```python
from build123d import *

# Parameters (mm, degrees)
EXTRUDE_THIN1_DEPTH = 635
FILLET1_R           = 1.27


with BuildPart() as part:
    # Sketch1 → Extrude-Thin1 (new body)
    with BuildSketch(Plane.XY):
        with BuildLine():
            Line((0, 0), (-15.875, 0))
            Line((-15.875, 0), (-15.875, 3.175))
            Line((-15.875, 3.175), (-19.05, 3.175))
            ThreePointArc((-19.05, 3.175), (-20.540376263, 7.805172974), (-24.451827217, 10.69658692))
            ThreePointArc((-24.451827217, 10.69658692), (-28.805679852, 14.276302994), (-29.685414913, 19.84375))
            Line((-29.685414913, 19.84375), (-32.860414913, 19.84375))
            Line((-32.860414913, 19.84375), (-32.860414913, 24.60625))
            Line((-32.860414913, 24.60625), (-36.494039614, 24.60625))
            ThreePointArc((-36.494039614, 24.60625), (-43.039469794, 22.912442068), (-47.941664913, 18.25625))
            Line((-47.941664913, 18.25625), (-56.672914913, 18.25625))
            Line((-56.672914913, 18.25625), (-56.672914913, 44.351036989))
            ThreePointArc((-56.672914913, 44.351036989), (-59.143520033, 43.316980719), (-60.876574207, 41.275))
            ThreePointArc((-60.876574207, 41.275), (-64.274926573, 48.035607826), (-63.5, 55.5625))
            Line((-63.5, 55.5625), (-34.925, 55.5625))
            Line((-34.925, 55.5625), (-34.925, 54.2925))
            Line((-34.925, 54.2925), (-62.614600616, 54.2925))
            ThreePointArc((-62.614600616, 54.2925), (-63.088488589, 48.638883567), (-60.958941974, 43.380273504))
            ThreePointArc((-60.958941974, 43.380273504), (-58.440775835, 45.159436942), (-55.402914913, 45.686679074))
            Line((-55.402914913, 45.686679074), (-55.402914913, 19.52625))
            Line((-55.402914913, 19.52625), (-48.62569758, 19.52625))
            ThreePointArc((-48.62569758, 19.52625), (-43.340564736, 24.19276788), (-36.494039614, 25.87625))
            Line((-36.494039614, 25.87625), (-31.590414913, 25.87625))
            Line((-31.590414913, 25.87625), (-31.590414913, 21.11375))
            Line((-31.590414913, 21.11375), (-27.922084416, 21.11375))
            ThreePointArc((-27.922084416, 21.11375), (-28.061990954, 15.63278224), (-24.046119572, 11.900040827))
            ThreePointArc((-24.046119572, 11.900040827), (-19.898030583, 9.05015784), (-17.868006799, 4.445))
            Line((-17.868006799, 4.445), (-14.605, 4.445))
            Line((-14.605, 4.445), (-14.605, 1.27))
            Line((-14.605, 1.27), (0, 1.27))
            Line((0, 1.27), (0, 0))
        make_face()
    extrude(amount=-EXTRUDE_THIN1_DEPTH)

    # Fillet1
    fillet1_edges = [part.edges().sort_by_distance(p)[0] for p in [
        (-55.402914913, 45.686679074, -317.5),
        (-31.590414913, 25.87625, -317.5),
        (-27.922084416, 21.11375, -317.5),
        (-14.605, 4.445, -317.5),
        (-15.875, 0, -317.5),
        (-19.05, 3.175, -317.5),
        (-32.860414913, 19.84375, -317.5),
        (-47.941664913, 18.25625, -317.5),
        (-56.672914913, 18.25625, -317.5),
        (-60.876574207, 41.275, -317.5),
        (-63.5, 55.5625, -317.5),
    ]]
    fillet(fillet1_edges, radius=FILLET1_R)


solid = part.part
```
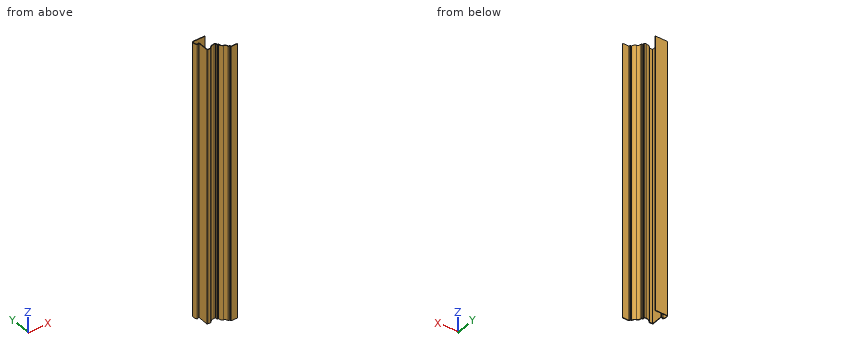
Check sheet for the modelled part. Datum: model origin and axes. Units: mm. Round coordinates to 2 decimals unless told otherwise and drop trailing zeros. Order: outer loops, then holes, each group sorted by start corner. A loop starts at its lowest first (then second) coordinate and runs counter-clockwise, first axis right, second up. Notation, with made-up numbers: (-14, 54) -> (39, 54) arc R13 cw to (39, 68) -> close; hole circle Ø6 at (2.5, -26.75). An arc over 180 degrees is marked (long way). One line per item, written item: value. Start each with the question number.
Q1. Thickness scan on line 1 (Y direction, x = -53.5, z = -240); line 2 (Y direction, x = -36, z = -183.5); line 3 (X direction, y = 21, z = -223). Record the ranges inside material, lowest first.
Q2. Gauge pin test, flat ends, axial feed: pin 1 Ø1 at (x, z) = (-31, -400.5) entering from -Y; pin 2 Ø4 at (x, z) = (-53, -228) entering from -Y; pin 3 Ø1.1 at (x, z) = (-34.5, -261.5) entering from -Y; pin 4 Ø2 at (x, y) = (-51, 22) entering from -Z. Record the tip position at first contact, or that the pin passes through.
Q3. Cross-section at B-B (x = -6). Record the boundary of the cut face in (y, z), and give its area (3 significant figures).
Q4. Cross-section at A-A (y = 32.5). Record the boundary of the cut face in (x, z).
Completed:
1. line 1: y = 18.26 to 19.53, 54.29 to 55.56
1. line 2: y = 24.61 to 25.88, 54.29 to 55.56
1. line 3: x = -56.67 to -55.4, -47.46 to -45.68, -32.86 to -29.16
2. pin 1: stops at y = 19.84
2. pin 2: stops at y = 18.26
2. pin 3: stops at y = 24.61
2. pin 4: passes through
3. outline: (0, -635) -> (1.27, -635) -> (1.27, 0) -> (0, 0) -> close
3. area: 806 mm²
4. outline: (-56.67, -635) -> (-55.4, -635) -> (-55.4, 0) -> (-56.67, 0) -> close
